from build123d import *

# Parameters (mm, degrees)
F1_DEPTH = 9
F2_W     = 6
F2_H     = 6
F3_DEPTH = 10


# Not quite as in the source:
# - a feature names something its author has since deleted; it is built from what else it names


with BuildPart() as f1:
    # F0 (on Top) → F1 (new body)
    with BuildSketch(Plane.XY):
        with BuildLine():
            Line((-25, -4.5), (0, -4.5))
            ThreePointArc((0, -4.5), (4.5, 0), (0, 4.5))
            Line((0, 4.5), (-25, 4.5))
            Line((-25, 4.5), (-25, 0))
            Line((-25, 0), (-25, -4.5))
        make_face()
        with BuildLine():
            ThreePointArc((3, 0), (0, -3), (-3, 0))
            ThreePointArc((-3, 0), (0, 3), (3, 0))
        make_face(mode=Mode.SUBTRACT)
    extrude(amount=F1_DEPTH)

    # F2 (on face) → F3 (cut)
    with BuildSketch(Plane(origin=(-25, 0, 0), x_dir=(0, -1, 0), z_dir=(-1, 0, 0))):
        with Locations((0, 4.5)):
            Rectangle(F2_W, F2_H)
    extrude(amount=-F3_DEPTH, mode=Mode.SUBTRACT)


solid = f1.part
The model under review builds one solid part; all positions refer to its coordinate system, in mm. A direction names the side the tool comes from. Round coordinates to 2 decimals unless told otherwise and drop trailing zeros. Order: outer loops, then holes, each group sorted by start corner. A loop starts at its lowest first (then second) coordinate and runs counter-clockwise, first axis right, second up. Notation, with made-up numbers: (-18, -38) -> (15, -38) arc R10 cw to (15, -23) -> close; hole circle Ø3 at (12, 45). An arc over 180 degrees is marked (long way). Return JSON: item names as keys, results as strings.
1. Take a section at A-A (x = -17.5). Write out the cut boundary in (y, z), then the cut area to 3 significant figures.
Answer block:
{"outline": "(-4.5, 0) -> (4.5, 0) -> (4.5, 9) -> (-4.5, 9) -> close; hole (-3, 1.5) -> (3, 1.5) -> (3, 7.5) -> (-3, 7.5) -> close", "area": "45.0 mm²"}
2. Take a section at B-B (z = 4.5). Write out the cut boundary in (x, y).
Answer block:
{"outline": "(-25, -4.5) -> (0, -4.5) arc R4.5 ccw to (0, 4.5) -> (-25, 4.5) -> (-25, 3) -> (-15, 3) -> (-15, -3) -> (-25, -3) -> close; hole circle Ø6 at (0, 0)"}
3. For L1, parallel to Y at x = 0, z = 2.5; L2, parallel to Z at x = -20, y = -1.25; L3, parallel to X at y = -2.75, z = 0.75, list the stretches that pass through material, from the lowest coordinate up. Write a range as [from, to].
Answer block:
{"L1": "y = [-4.5, -3], [3, 4.5]", "L2": "z = [0, 1.5], [7.5, 9]", "L3": "x = [-25, -1.2], [1.2, 3.56]"}
4. Take a section at C-C (y = 0). Write out the cut boundary in (x, z), then the cut area to 4 significant figures.
Answer block:
{"outline": "(-25, 0) -> (-3, 0) -> (-3, 9) -> (-25, 9) -> (-25, 7.5) -> (-15, 7.5) -> (-15, 1.5) -> (-25, 1.5) -> close; (3, 0) -> (4.5, 0) -> (4.5, 9) -> (3, 9) -> close", "area": "151.5 mm²"}
5. For faces 4 (the face through (-20, -3, 4)), 5 (the face through (-10, 0, 0)), list the 3-axis set-ups (+Z, -Z, +X, -X, +Y, -Y) from which the entire face can be reached by the end or side of a thin tool; tool diameter is ignored.
Answer block:
{"face 4": "-X", "face 5": "-Z, +X, -X, +Y, -Y"}
6. Take a section at D-D (x = -2). Write out the cut boundary in (y, z), then the cut area to 3 significant figures.
Answer block:
{"outline": "(-4.5, 0) -> (-2.24, 0) -> (-2.24, 9) -> (-4.5, 9) -> close; (2.24, 0) -> (4.5, 0) -> (4.5, 9) -> (2.24, 9) -> close", "area": "40.8 mm²"}
7. The part is to be moulded in two halves that separate along Y. For faces 1 (the face through (-20, 0, 7.5)), 2 (the face through (-12, 4.5, 4)), 3 (the face through (4.5, -0.1, 4.4)), say which applies: +Y half, -Y half, draft (parallel to the pull), parting line (faces both ways), or undercut.
Answer block:
{"face 1": "undercut", "face 2": "+Y half", "face 3": "parting line"}
